Input: part model. Units: mm. Frame: model coordinates. A direction names the side the tool comes from. Round coordinates to 2 decimals unless told otherwise and drop trailing zeros. Loops run counter-clockwise (first coordinate to the right, second up) from the corner with the lowest first, then second, coordinate; pieces in that order, holes last.
1) Ray query, line 1 along Y through (x, z) = (-1.25, -1.25); line 2 along X through (y, z) = (7, 0.25); line 3 along Z through (x, y) = (-0.75, -0.5). Return the intervals inside material, ascending.
2) Section D-D, the plane x = 3. Return loops of the section in (y, z), and give its area (3 significant figures).
3) Section C-C, the plane z = 3.25. Return loops of the section in (x, y), and give its area (3 significant figures).
4) Section A-A, the plane x = 0. Return loops of the section in (y, z) (3 decimals), and give its area (3 significant figures).
5) First-contact query: pin 1 (3 mm diameter, centred on y = -8.5, z = 2.5, fed in from +X); pin 2 (1 mm diameter, centred on y = -9, z = 0, fed in from +X); pin 3 (3 mm diameter, centred on x = -1.5, y = 15, fed in from -Z). Flat tips, straight axial feed; report the tip coordinate or a pass-through.
6) Section B-B, the plane y = -5. Return loops of the section in (x, z), and give its area (3 significant figures).
7) Access query for faces 1 (the face through (0, 0, -2)), 2 (the face through (0.45, 12.76, 1.43)), 3 (the face through (0, 1, 4.5)). Directions: +Z, -Z, +X, -X, +Y, -Y. A direction counts if a zero-diameter tool reaches every point of the face in a straight line with its end or side. Return the directions, or none.
from build123d import *

# Parameters (mm, degrees)
SKETCH1_R           = 1.5
BOSS_EXTRUDE1_DEPTH = 23.825
BOSS_EXTRUDE2_DEPTH = 2
BOSS_EXTRUDE3_START = 20.8
SKETCH4_R           = 1.5
BOSS_EXTRUDE3_DEPTH = 20.8


with BuildPart() as part:
    # Sketch1 → Boss-Extrude1 (new body)
    with BuildSketch(Plane(origin=(0, 0, 0), x_dir=(1, 0, 0), z_dir=(0, 1, 0))):
        with Locations(Location((0, 0, 0), (0, 0, 270))):
            Circle(SKETCH1_R)
    extrude(amount=BOSS_EXTRUDE1_DEPTH)

    # Sketch3 → Boss-Extrude2 (add)
    with BuildSketch(Plane(origin=(0, 0, 0), x_dir=(-1, 0, 0), z_dir=(0, -1, 0))):
        Polygon((5.196152423, 0), (2.598076211, 4.5), (-2.598076211, 4.5), (-5.196152423, 0), (-2.598076211, -4.5), (2.598076211, -4.5), align=None)
    extrude(amount=-BOSS_EXTRUDE2_DEPTH)

    # Sketch4 → Boss-Extrude3 (add)
    with BuildSketch(Plane(origin=(0, 0, 0), x_dir=(-1, 0, 0), z_dir=(0, -1, 0)).offset(BOSS_EXTRUDE3_START)):
        with Locations(Location((0, 0, 0), (0, 0, 90))):
            Circle(SKETCH4_R)
    extrude(amount=-BOSS_EXTRUDE3_DEPTH)


solid = part.part
Final values:
1. line 1: y = 0 to 2
1. line 2: x = -1.48 to 1.48
1. line 3: z = -1.3 to 1.3
2. outline: (0, -3.8) - (2, -3.8) - (2, 3.8) - (0, 3.8) - close
2. area: 15.2 mm2
3. outline: (-3.32, 0) - (3.32, 0) - (3.32, 2) - (-3.32, 2) - close
3. area: 13.3 mm2
4. outline: (-20.8, -1.5) - (0, -1.5) - (0, -4.5) - (2, -4.5) - (2, -1.5) - (23.825, -1.5) - (23.825, 1.5) - (2, 1.5) - (2, 4.5) - (0, 4.5) - (0, 1.5) - (-20.8, 1.5) - close
4. area: 146 mm2
5. pin 1: stops at x = 1.12
5. pin 2: stops at x = 1.5
5. pin 3: stops at z = -1.5
6. outline: circle Ø3 at (0, 0)
6. area: 7.07 mm2
7. face 1: -Y
7. face 2: +Y
7. face 3: +Z, +X, -X, +Y, -Y
